from build123d import *

# Parameters (mm, degrees)
SKETCH1_W                      = 25
SKETCH1_H                      = 38.2
BASE_FLANGE1_DEPTH             = 1.5
EDGE_FLANGE1_STRIP_W           = 9.3
EDGE_FLANGE1_STRIP_H           = 1.5
EDGE_FLANGE1_STRIP_CUT_DEPTH   = 25
EDGE_FLANGE1_STRIP_2_W         = 9.3
EDGE_FLANGE1_STRIP_2_H         = 1.5
EDGE_FLANGE1_STRIP_CUT_2_DEPTH = 25
EDGE_FLANGE1_DEPTH             = 25
EDGE_FLANGE1_BEND_DEPTH        = 25
CUT_EXTRUDE1_REACH             = 57.803
SKETCH12_R                     = 1.5
SKETCH12_R_2                   = 3.25
CUT_EXTRUDE2_REACH             = 57.803
SKETCH13_R                     = 4
SKETCH13_R_2                   = 1.1
FILLET1_R                      = 12.5
SKETCH14_R                     = 1.6
TAB1_DEPTH                     = 1.5


# Sheet-metal steps are written as plain solids
with BuildPart() as part:
    # Sketch1 → Base-Flange1 (new body)
    with BuildSketch(Plane(origin=(0, 0, 0), x_dir=(1, 0, 0), z_dir=(0, 1, 0))):
        Rectangle(SKETCH1_W, SKETCH1_H)
    extrude(amount=-BASE_FLANGE1_DEPTH)

    # Edge-Flange1 strip (across the edge) → Edge-Flange1 strip cut (cut)
    with BuildSketch(Plane(origin=(12.5, -1.5, 19.1), x_dir=(0, 0, -1), z_dir=(-1, 0, 0))):
        with Locations((-3, -0.75)):
            Rectangle(EDGE_FLANGE1_STRIP_W, EDGE_FLANGE1_STRIP_H)
    extrude(amount=EDGE_FLANGE1_STRIP_CUT_DEPTH, mode=Mode.SUBTRACT)

    # Edge-Flange1 strip 2 (across the edge) → Edge-Flange1 strip cut 2 (cut)
    with BuildSketch(Plane(origin=(-12.5, -1.5, -19.1), x_dir=(0, 0, 1), z_dir=(1, 0, 0))):
        with Locations((-3, -0.75)):
            Rectangle(EDGE_FLANGE1_STRIP_2_W, EDGE_FLANGE1_STRIP_2_H)
    extrude(amount=EDGE_FLANGE1_STRIP_CUT_2_DEPTH, mode=Mode.SUBTRACT)

    # Edge-Flange1 section (across the edge) → Edge-Flange1 (add)
    with BuildSketch(Plane(origin=(12.5, -1.5, 19.1), x_dir=(0, 0, -1), z_dir=(-1, 0, 0))):
        with BuildLine():
            Line((-1.5, 1.65), (-1.5, 34))
            Line((-1.5, 34), (0, 34))
            Line((0, 34), (0, 1.65))
            ThreePointArc((0, 1.65), (0.483273811, 0.483273811), (1.65, 0))
            Line((1.65, 0), (1.65, -1.5))
            ThreePointArc((1.65, -1.5), (-0.577386361, -0.577386361), (-1.5, 1.65))
        make_face()
    extrude(amount=EDGE_FLANGE1_DEPTH)

    # Edge-Flange1 section 2 (across the edge) → Edge-Flange1 bend (add)
    with BuildSketch(Plane(origin=(-12.5, -1.5, -19.1), x_dir=(0, 0, 1), z_dir=(1, 0, 0))):
        with BuildLine():
            Line((-1.5, 1.65), (-1.5, 34))
            Line((-1.5, 34), (0, 34))
            Line((0, 34), (0, 1.65))
            ThreePointArc((0, 1.65), (0.483273811, 0.483273811), (1.65, 0))
            Line((1.65, 0), (1.65, -1.5))
            ThreePointArc((1.65, -1.5), (-0.577386361, -0.577386361), (-1.5, 1.65))
        make_face()
    extrude(amount=EDGE_FLANGE1_BEND_DEPTH)

    # Sketch12 → Cut-Extrude1 (cut, up to next)
    with BuildSketch(Plane.XY.offset(20.6), mode=Mode.PRIVATE) as cut_extrude1_sk1:
        with Locations((-4.949747468, -18.050252532)):
            Circle(SKETCH12_R)
    cut_extrude1_tool1 = extrude(cut_extrude1_sk1.sketch, amount=-CUT_EXTRUDE1_REACH, mode=Mode.PRIVATE) & part.part
    # Sketch12 → Cut-Extrude1 (cut, up to next)
    with BuildSketch(Plane.XY.offset(20.6), mode=Mode.PRIVATE) as cut_extrude1_sk2:
        with Locations((4.949747468, -18.050252532)):
            Circle(SKETCH12_R)
    cut_extrude1_tool2 = extrude(cut_extrude1_sk2.sketch, amount=-CUT_EXTRUDE1_REACH, mode=Mode.PRIVATE) & part.part
    # Sketch12 → Cut-Extrude1 (cut, up to next)
    with BuildSketch(Plane.XY.offset(20.6), mode=Mode.PRIVATE) as cut_extrude1_sk3:
        with Locations((-4.949747468, -27.949747468)):
            Circle(SKETCH12_R)
    cut_extrude1_tool3 = extrude(cut_extrude1_sk3.sketch, amount=-CUT_EXTRUDE1_REACH, mode=Mode.PRIVATE) & part.part
    # Sketch12 → Cut-Extrude1 (cut, up to next)
    with BuildSketch(Plane.XY.offset(20.6), mode=Mode.PRIVATE) as cut_extrude1_sk4:
        with Locations((4.949747468, -27.949747468)):
            Circle(SKETCH12_R)
    cut_extrude1_tool4 = extrude(cut_extrude1_sk4.sketch, amount=-CUT_EXTRUDE1_REACH, mode=Mode.PRIVATE) & part.part
    # Sketch12 → Cut-Extrude1 (cut, up to next)
    with BuildSketch(Plane.XY.offset(20.6), mode=Mode.PRIVATE) as cut_extrude1_sk5:
        with Locations((0, -23)):
            Circle(SKETCH12_R_2)
    cut_extrude1_tool5 = extrude(cut_extrude1_sk5.sketch, amount=-CUT_EXTRUDE1_REACH, mode=Mode.PRIVATE) & part.part
    add(cut_extrude1_tool1.solids().sort_by_distance((-4.949747, -18.050253, 20.6))[0], mode=Mode.SUBTRACT)
    add(cut_extrude1_tool2.solids().sort_by_distance((4.949747, -18.050253, 20.6))[0], mode=Mode.SUBTRACT)
    add(cut_extrude1_tool3.solids().sort_by_distance((-4.949747, -27.949747, 20.6))[0], mode=Mode.SUBTRACT)
    add(cut_extrude1_tool4.solids().sort_by_distance((4.949747, -27.949747, 20.6))[0], mode=Mode.SUBTRACT)
    add(cut_extrude1_tool5.solids().sort_by_distance((0, -23, 20.6))[0], mode=Mode.SUBTRACT)

    # Sketch13 → Cut-Extrude2 (cut, up to next)
    with BuildSketch(Plane(origin=(0, 0, -20.6), x_dir=(-1, 0, 0), z_dir=(0, 0, -1)), mode=Mode.PRIVATE) as cut_extrude2_sk1:
        with Locations(Location((0, -23, 0), (0, 0, 90))):
            Circle(SKETCH13_R)
    cut_extrude2_tool1 = extrude(cut_extrude2_sk1.sketch, amount=-CUT_EXTRUDE2_REACH, mode=Mode.PRIVATE) & part.part
    # Sketch13 → Cut-Extrude2 (cut, up to next)
    with BuildSketch(Plane(origin=(0, 0, -20.6), x_dir=(-1, 0, 0), z_dir=(0, 0, -1)), mode=Mode.PRIVATE) as cut_extrude2_sk2:
        with Locations(Location((0, -30, 0), (0, 0, 90))):
            Circle(SKETCH13_R_2)
    cut_extrude2_tool2 = extrude(cut_extrude2_sk2.sketch, amount=-CUT_EXTRUDE2_REACH, mode=Mode.PRIVATE) & part.part
    # Sketch13 → Cut-Extrude2 (cut, up to next)
    with BuildSketch(Plane(origin=(0, 0, -20.6), x_dir=(-1, 0, 0), z_dir=(0, 0, -1)), mode=Mode.PRIVATE) as cut_extrude2_sk3:
        with Locations(Location((-7, -23, 0), (0, 0, 90))):
            Circle(SKETCH13_R_2)
    cut_extrude2_tool3 = extrude(cut_extrude2_sk3.sketch, amount=-CUT_EXTRUDE2_REACH, mode=Mode.PRIVATE) & part.part
    # Sketch13 → Cut-Extrude2 (cut, up to next)
    with BuildSketch(Plane(origin=(0, 0, -20.6), x_dir=(-1, 0, 0), z_dir=(0, 0, -1)), mode=Mode.PRIVATE) as cut_extrude2_sk4:
        with Locations(Location((0, -16, 0), (0, 0, 90))):
            Circle(SKETCH13_R_2)
    cut_extrude2_tool4 = extrude(cut_extrude2_sk4.sketch, amount=-CUT_EXTRUDE2_REACH, mode=Mode.PRIVATE) & part.part
    # Sketch13 → Cut-Extrude2 (cut, up to next)
    with BuildSketch(Plane(origin=(0, 0, -20.6), x_dir=(-1, 0, 0), z_dir=(0, 0, -1)), mode=Mode.PRIVATE) as cut_extrude2_sk5:
        with Locations(Location((7, -23, 0), (0, 0, 90))):
            Circle(SKETCH13_R_2)
    cut_extrude2_tool5 = extrude(cut_extrude2_sk5.sketch, amount=-CUT_EXTRUDE2_REACH, mode=Mode.PRIVATE) & part.part
    add(cut_extrude2_tool1.solids().sort_by_distance((0, -23, -20.6))[0], mode=Mode.SUBTRACT)
    add(cut_extrude2_tool2.solids().sort_by_distance((0, -30, -20.6))[0], mode=Mode.SUBTRACT)
    add(cut_extrude2_tool3.solids().sort_by_distance((7, -23, -20.6))[0], mode=Mode.SUBTRACT)
    add(cut_extrude2_tool4.solids().sort_by_distance((0, -16, -20.6))[0], mode=Mode.SUBTRACT)
    add(cut_extrude2_tool5.solids().sort_by_distance((-7, -23, -20.6))[0], mode=Mode.SUBTRACT)

    # Fillet1
    fillet1_edges = [part.edges().sort_by_distance(p)[0] for p in [
        (12.5, -35.5, 19.85),
        (-12.5, -35.5, 19.85),
        (-12.5, -35.5, -19.85),
        (12.5, -35.5, -19.85),
    ]]
    fillet(fillet1_edges, radius=FILLET1_R - 0.0001)  # a hair under: the kernel refuses the full size

    # Sketch14 → Tab1 (add)
    with BuildSketch(Plane.XZ.offset(1.5)):
        with BuildLine():
            Line((12.5, -5.581701947), (12.5, 5.581701947))
            ThreePointArc((12.5, 5.581701947), (13.935678731, 4.66460431), (15.532990604, 4.072289972))
            ThreePointArc((15.532990604, 4.072289972), (18.701263524, 0), (15.532990604, -4.072289972))
            ThreePointArc((15.532990604, -4.072289972), (13.935678731, -4.66460431), (12.5, -5.581701947))
        make_face()
        with Locations(Location((14.5, 0, 0), (0, 0, 270))):
            Circle(SKETCH14_R, mode=Mode.SUBTRACT)
    extrude(amount=-TAB1_DEPTH)


solid = part.part
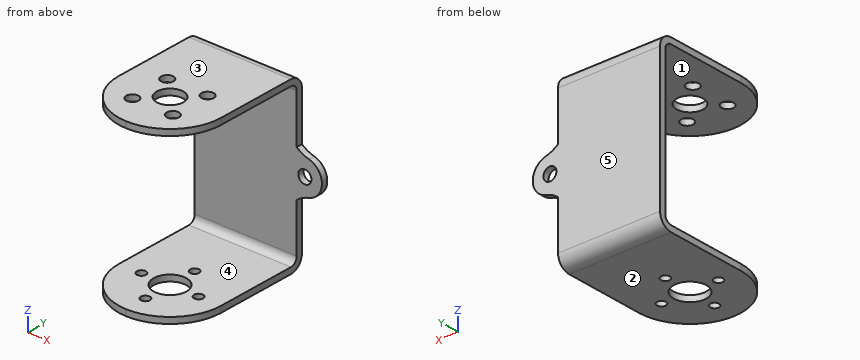
The listing builds one solid part. Answer for the finished solid, in the listing's coordinates (mm). Face numbers are marked on the shaded views. A direction names the side the tool comes from. Give positions to 0.01 mm unless a question says otherwise; leave off trailing zeros. Loops run counter-clockwise (first coordinate to the right, second up) from the corner with the lowest first, then second, coordinate; pieces in that order, holes last. Notation, with made-up numbers: (-27, 68.25) - (19, 68.25) arc R26 cw to (19, 107.25) - close; hole circle Ø11 at (-13, 17.5). An arc over 180 degrees is marked (long way). Answer as a JSON object with one key per item and string values.
1. Find the intervals of material crossed by L1, parallel to Z at x = -4.5, y = -10; L2, parallel to Y at x = -9, z = 10; L3, parallel to Y at x = 1, z = 19.5, in increasing order. Write a range as [from, to].
Determined:
{"L1": "[-20.6, -19.1], [19.1, 20.6]", "L2": "[-1.5, 0]", "L3": "[-35.46, -26.09], [-19.91, -0.76]"}
2. Flat-ended cylindrical pins translate along their axes: pin 1 Ø1 at (x, z) = (5.5, 15.5) entering from -Y; pin 2 Ø12 at (x, y) = (-5.5, -19) entering from +Z; pin 3 Ø7.5 at (y, z) = (-9, -16) entering from +X; pin 4 Ø2.5 at (x, y) = (4.95, -18.05) entering from +Z. Find the tip coordinate at first contact, or state that the pin passes through.
Determined:
{"pin 1": "y = -1.5", "pin 2": "z = 20.6", "pin 3": "x = 12.5", "pin 4": "z = -19.1"}
3. For a pull along Z with two mould halves and no side action, classify the marked faces 3, 4 and 5 as pulls with the +Z half, pulls with the -Z half, needs draft (parallel to the pull), parting line crosses it, or undercut.
Determined:
{"face 3": "pulls with the +Z half", "face 4": "undercut", "face 5": "needs draft"}
4. For the marked faces 1 and 2, determine the directions among +Z, -Z, +X, -X, +Y, -Y from which every point of the face is accessible in a straight line to the end or side of a thin tool.
Determined:
{"face 1": "+X, -X, -Y", "face 2": "-Z, +X, -X, +Y, -Y"}
5. A cutting plane is placed at C-C (x = -7). Write down the section's boundary in (y, z), then the cut area to 3 significant figures.
Determined:
{"outline": "(-33.36, -20.6) - (-24.1, -20.6) - (-24.1, -19.1) - (-33.36, -19.1) - close; (-33.36, 19.1) - (-3.15, 19.1) arc R1.65 cw to (-1.5, 17.45) - (-1.5, -17.45) arc R1.65 cw to (-3.15, -19.1) - (-21.9, -19.1) - (-21.9, -20.6) - (-3.15, -20.6) arc R3.15 ccw to (0, -17.45) - (0, 17.45) arc R3.15 ccw to (-3.15, 20.6) - (-33.36, 20.6) - close", "area": "151 mm²"}
6. A cutting plane is placed at D-D (y = -5). Write down the section's boundary in (x, z), then the cut area to 3 significant figures.
Determined:
{"outline": "(-12.5, -20.6) - (12.5, -20.6) - (12.5, -19.1) - (-12.5, -19.1) - close; (-12.5, 19.1) - (12.5, 19.1) - (12.5, 20.6) - (-12.5, 20.6) - close", "area": "75.0 mm²"}
7. A cutting plane is placed at A-A (z = 0). Write down the section's boundary in (x, y).
Determined:
{"outline": "(-12.5, -1.5) - (12.9, -1.5) - (12.9, 0) - (-12.5, 0) - close; (16.1, -1.5) - (18.7, -1.5) - (18.7, 0) - (16.1, 0) - close"}
8. A cutting plane is placed at B-B (y = -16). Write down the section's boundary in (x, z).
Determined:
{"outline": "(-12.5, -20.6) - (-1.1, -20.6) - (-1.1, -19.1) - (-12.5, -19.1) - close; (-12.5, 19.1) - (12.5, 19.1) - (12.5, 20.6) - (-12.5, 20.6) - close; (1.1, -20.6) - (12.5, -20.6) - (12.5, -19.1) - (1.1, -19.1) - close"}
